CAD build for the part. Positions are in the model's coordinates, mm. Coordinates: 2 decimals unless noted, no trailing zeros. Loops run counter-clockwise (first coordinate to the right, second up) from the corner with the lowest first, then second, coordinate; pieces in that order, holes last. Notation, with made-up numbers: (66, -20) - (112, -20) arc R26 ccw to (112, -1) - close; hole circle Ø2 at (48.5, 13). An arc over 180 degrees is marked (long way). Put each result on its own line as item: value.
Autodesk Inventor part; units mm, degrees
ref_plane "YZ Plane" through (0, 0, 0) normal (1, 0, 0) x (0, 1, 0)
ref_plane "XZ Plane" through (0, 0, 0) normal (0, 1, 0) x (-1, 0, 0)
ref_plane "XY Plane" through (0, 0, 0) normal (0, 0, 1) x (1, 0, 0)
sketch "Sketch1" plane through (0, 0, 0) normal (0, 1, 0) x (-1, 0, 0)
  circle A0 centre (0, 0) radius 9.5
  dimension "d0" = 19
extrude "Extrusion1" add sketch "Sketch1" along normal blind 15 draft -10
fillet "Fillet1" radius 2 1 edges at (6.8551, 15, 0)
fillet "Fillet2" radius 0.5 1 edges at (9.5, 0, 0)
sketch "Sketch2" plane through (0, 0, 0) normal (0, -1, 0) x (1, 0, 0)
  circle A0 centre (0, 0) radius 2
  dimension "d5" = 4
extrude "Extrusion2" cut sketch "Sketch2" against normal blind 15
sketch "Sketch3" plane through (0, 15, 0) normal (0, 1, 0) x (1, 0, 0)
  circle A0 centre (0, 0) radius 5
  dimension "d8" = 10
extrude "Extrusion3" cut sketch "Sketch3" against normal blind 7
fillet "Fillet3" radius 1 1 edges at (-5, 8, 0)
properties part number "Patas_para_licuadora" material "Rubber"
Q1. Pin check, flat tips, straight feed: pin 1 Ø1.5 at (x, y) = (-3, 7) entering from -Z; pin 2 Ø4 at (x, z) = (-2, 1.5) entering from +Y; pin 3 Ø2 at (x, y) = (-3.5, 12.5) entering from -Z; pin 4 Ø3.5 at (x, z) = (0, 0) entering from -Y. Stop position of each tip, or through.
Determined:
pin 1: z = -7.99
pin 2: y = 8.13
pin 3: z = -6.9
pin 4: through
Q2. Slice it at C-C, the plane y = 6.75. Give the cut face in (x, z).
Determined:
outline: circle Ø16.62 at (0, 0); hole circle Ø4 at (0, 0)
Q3. Slice it at B-B, the plane y = 5.25. Give the cut face in (x, z).
Determined:
outline: circle Ø17.15 at (0, 0); hole circle Ø4 at (0, 0)
Q4. Slice it at A-A, the plane x = 0. Give the cut face in (y, z).
Determined:
outline: (0, -8.9) arc R0.5 ccw to (0.59, -9.4) - (13.35, -7.15) arc R2 ccw to (15, -5.18) - (15, -5) - (9, -5) arc R1 cw to (8, -4) - (8, -2) - (0, -2) - close; (0, 2) - (8, 2) - (8, 4) arc R1 cw to (9, 5) - (15, 5) - (15, 5.18) arc R2 ccw to (13.35, 7.15) - (0.59, 9.4) arc R0.5 ccw to (0, 8.9) - close
Q5. Wall check: L1, parallel to Z at x = 0, y = 5.25; L2, parallel to Z at x = 0, y = 13.75; L3, parallel to X at y = 11.5, z = 1.25. Give the ranges that are in metal, low to high. Write a range as from..to.
Determined:
L1: -8.57..-2, 2..8.57
L2: -7.03..-5, 5..7.03
L3: -7.37..-4.84, 4.84..7.37
Q6. Mould opens along Z. For faces 1 (the flat face through (-2, 8, 1)), 2 (the conical face through (-7.666, 8.296, -2.414)), 3 (the cylindrical face through (0, 4, -2)), 4 (the flat face through (-2, 0, -2)) say: +Z half, -Z half, draft (parallel to the pull), parting line (faces both ways), or undercut.
Determined:
face 1: undercut
face 2: parting line
face 3: undercut
face 4: draft
